Could you check a few things on this model? Use its own coordinates, in mm. Face numbers are marked on the shaded views. Give positions to 0.01 mm unless a question says otherwise; leave off trailing zeros. Loops run counter-clockwise (first coordinate to the right, second up) from the corner with the lowest first, then second, coordinate; pieces in that order, holes last. Notation, with made-up numbers: M -0.5,18 L 49.5,18 A17 ccw 49.5,35 Z; hole C -14,-21.75 d6. An arc over 180 degrees is marked long. Return JSON: item names as keys, results as strings. Group by question number.
1. Please list where these lines run through material, in increasing order: line 1 (X direction, y = -1, z = 0); line 2 (Z direction, x = 0, y = -2.25).
2. If we section it at D-D (x = 3.75): Write out the boundary of the cut face in (y, z).
3. For pin 1 (1.5 mm diameter, centred on y = -2, z = 2.5, fed in from +X), with a flat end and sliding along its axis, tell me the tip position at first contact or that it passes through.
4. If we mould it in two halves opening along Z, with no side actions, what happens to the marked faces 1, 2, 3 and 4? For each: +Z half, -Z half, draft (parallel to the pull), parting line (faces both ways), or undercut.
5. If we section it at C-C (y = -1.75): Write out the boundary of the cut face in (x, z), plus the area to 3 significant figures.
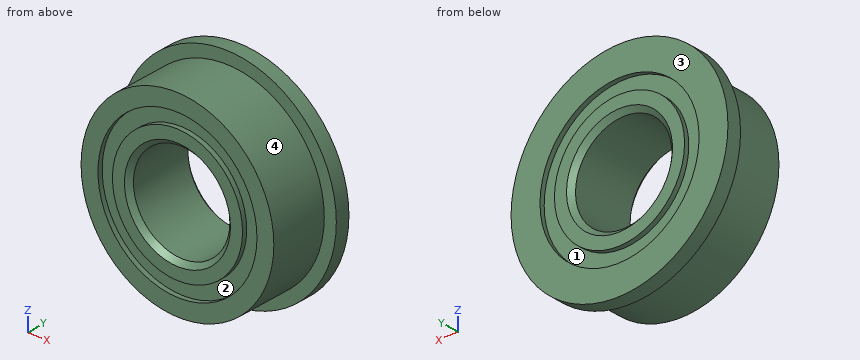
```python
from build123d import *

# Parameters (mm, degrees)
CHAMFER1_SIZE = 0.2


with BuildPart() as part:
    # Sketch1 → Revolve1 (revolve)
    with BuildSketch(Plane.XY):
        Polygon((2, -2.4), (2, 0.6), (2.7, 0.6), (2.7, 0.4), (3.3, 0.4), (3.3, 0.6), (4.5, 0.6), (4.5, 0), (4, 0), (4, -2.4), (3.3, -2.4), (3.3, -2.2), (2.7, -2.2), (2.7, -2.4), align=None)
    revolve(axis=Axis((0, 0, 0), (0, 1, 0)))

    # Chamfer1
    chamfer1_edges = [part.edges().sort_by_distance(p)[0] for p in [
        (-2, -2.4, 0),
        (-2, 0.6, 0),
    ]]
    chamfer(chamfer1_edges, length=CHAMFER1_SIZE)


solid = part.part
```
Answer:
{
 "1": {"line 1": "x = -4 to -2, 2 to 4", "line 2": "z = -4 to -3.3, -2.7 to -2.05, 2.05 to 2.7, 3.3 to 4"},
 "2": {"outline": "M -2.4,-1.39 L 0,-1.39 L 0,-2.49 L 0.6,-2.49 L 0.6,2.49 L 0,2.49 L 0,1.39 L -2.4,1.39 Z"},
 "3": {"pin 1": "stops at x = 3.6"},
 "4": {"face 1": "undercut", "face 2": "undercut", "face 3": "draft", "face 4": "parting line"},
 "5": {"outline": "C 0,0 d8; hole C 0,0 d4", "area": "37.7 mm²"}
}
